Model file for the job. Use its own axes, mm. A direction names the side the tool comes from. Round coordinates to 2 decimals unless told otherwise and drop trailing zeros. Order: outer loops, then holes, each group sorted by start corner. A loop starts at its lowest first (then second) coordinate and runs counter-clockwise, first axis right, second up. Notation, with made-up numbers: M 76.25,30 L 94.25,30 A33 ccw 94.25,69 Z; hole C -32,63 d1. An arc over 180 degrees is marked long. Return JSON: item names as keys, results as strings. Group by question number.
Item 1: Pin check, flat tips, straight feed: pin 1 Ø13 at (x, y) = (18, -36.5) entering from +Z; pin 2 Ø1.5 at (x, z) = (29.5, 12) entering from -Y (3 decimals); pin 3 Ø8 at (x, y) = (10.5, 11) entering from +Z. Stop position of each tip, or through.
Item 2: Slice it at B-B on z = -6. Write the cut outline in (x, y) (3 decimals), then the cut area to 3 significant figures.
Item 3: Pull direction Y, two halves, no side cores. Call faces 4 (the face through (-45.12, -25.07, 6.59)), 5 (the face through (-15, 36.875, -2)), 6 (the face through (-44.425, 8, 9)): pulls with the +Y half, pulls with the -Y half, needs draft (parallel to the pull), parting line crosses it, or undercut.
Item 4: Probe line 1 along X through (y, z) = (34, -4) (3 decimals); line 2 along Z through (x, y) = (-12.5, -16); line 3 along Z through (x, y) = (-10.5, -0.5). List the from-to ranges inside material, lowest first.
Item 5: Slice it at D-D on x = -9. Write the cut outline in (y, z) (3 decimals).
Item 6: Slice it at A-A on y = 7. Write the cut outline in (x, z) (3 decimals), then the cut area to 3 significant figures.
Item 7: Slice it at C-C on x = -31. Write the cut outline in (y, z) (3 decimals).
Item 8: Which spindle directions (+Z, -Z, +X, -X, +Y, -Y) get a long thin tool onto all of the face, cutting with end or side? Do faces 1 (the face through (-42, 29.375, 9)), 2 (the face through (-37, -5.425, -1)), 3 (the face through (21.39, -40.7, 6.28)). Say none if no direction does.
from build123d import *

# Parameters (mm, degrees)
SKETCH1_W                             = 92.75
SKETCH1_H                             = 86.75
SKETCH1_R                             = 1.55
BOSS_EXTRUDE1_FIRST_PCB_DEPTH         = 1.6
SKETCH2_R                             = 6
BOSS_EXTRUDE2_SPEAKER_DEPTH           = 9.5
SKETCH15_R                            = 1.25
CUT_EXTRUDE1_SPEAKER_HOLE_DEPTH       = 5
SKETCH3_W                             = 12
SKETCH3_H                             = 11.65
BOSS_EXTRUDE3_ROTARY_SWITCH_DEPTH     = 4.5
SKETCH4_W                             = 5.83
SKETCH4_H                             = 5.83
BOSS_EXTRUDE4_RESET_SWITCH_DEPTH      = 3.5
SKETCH5_R                             = 1.75
BOSS_EXTRUDE5_RESET_BUTTON_DEPTH      = 0.5
SKETCH16_R                            = 3.415
BOSS_EXTRUDE6_ROTARY_SWITCH_DEPTH     = 7
SKETCH17_R                            = 2.935
BOSS_EXTRUDE7_ROTARY_SWITCH_DEPTH     = 6.4
BOSS_EXTRUDE8_ROTARY_SWITCH_DEPTH     = 6.2
BOSS_EXTRUDE9_SD_CARD_SLOT_DEPTH      = 3
SKETCH19_W                            = 50
SKETCH19_H                            = 2.5
BOSS_EXTRUDE10_CONNECTOR_DEPTH        = 4.2
SKETCH11_W                            = 92.75
SKETCH11_H                            = 70
SKETCH11_R                            = 1.55
BOSS_EXTRUDE11_UPPER_PCB_DEPTH        = 1.6
SKETCH12_W                            = 78.45
SKETCH12_H                            = 51
BOSS_EXTRUDE12_LCD_DEPTH              = 8.3
SKETCH24_W                            = 5.4
SKETCH24_H                            = 43
BOSS_EXTRUDE13_LCD_BUMPOUT_DEPTH      = 3.5
CUT_EXTRUDE2_SCREEN_RECESS_DEPTH      = 1
SKETCH21_W                            = 20.2
SKETCH21_H                            = 8.85
SKETCH21_W_2                          = 18.2
SKETCH21_H_2                          = 6.85
BOSS_EXTRUDE14_CONNECTORS_DEPTH       = 9
SKETCH22_W                            = 18.2
SKETCH22_H                            = 6.85
BOSS_EXTRUDE15_CONNECTOR_RECESS_DEPTH = 2.55
SKETCH23_W                            = 4.4
SKETCH23_H                            = 1
CUT_EXTRUDE3_CONNECTOR_NOTCH_DEPTH    = 6.45
SKETCH20_W                            = 2.153
SKETCH20_H                            = 23.75
BOSS_EXTRUDE16_SD_CARD_DEPTH          = 10.4
FILLET1_SD_CARD_R                     = 1


with BuildPart() as part:
    # Sketch1 → Boss-Extrude1 - First PCB (new body)
    with BuildSketch(Plane.XY):
        Rectangle(SKETCH1_W, SKETCH1_H)
        with Locations((-43.975, 40.975)):
            Circle(SKETCH1_R, mode=Mode.SUBTRACT)
        with Locations((43.975, 40.975)):
            Circle(SKETCH1_R, mode=Mode.SUBTRACT)
        with Locations((43.975, -24.025)):
            Circle(SKETCH1_R, mode=Mode.SUBTRACT)
        with Locations((-43.975, -24.025)):
            Circle(SKETCH1_R, mode=Mode.SUBTRACT)
    extrude(amount=BOSS_EXTRUDE1_FIRST_PCB_DEPTH)

    # Sketch2 → Boss-Extrude2 - Speaker (add)
    with BuildSketch(Plane.XY.offset(1.6)):
        with Locations((18.625, -35.375)):
            Circle(SKETCH2_R)
    extrude(amount=BOSS_EXTRUDE2_SPEAKER_DEPTH)

    # Sketch15 → Cut-Extrude1 - Speaker Hole (cut)
    with BuildSketch(Plane.XY.offset(11.1)):
        with Locations((18.625, -35.375)):
            Circle(SKETCH15_R)
    extrude(amount=-CUT_EXTRUDE1_SPEAKER_HOLE_DEPTH, mode=Mode.SUBTRACT)

    # Sketch3 → Boss-Extrude3 - Rotary Switch (add)
    with BuildSketch(Plane(origin=(0, 0, 1.6), x_dir=(-1, 0, 0), z_dir=(0, 0, 1))):
        with Locations((-36.375, 35.375)):
            Rectangle(SKETCH3_W, SKETCH3_H)
    extrude(amount=BOSS_EXTRUDE3_ROTARY_SWITCH_DEPTH)

    # Sketch4 → Boss-Extrude4 - Reset Switch (add)
    with BuildSketch(Plane(origin=(0, 0, 1.6), x_dir=(-1, 0, 0), z_dir=(0, 0, 1))):
        with Locations((-3.375, 35.375)):
            Rectangle(SKETCH4_W, SKETCH4_H)
    extrude(amount=BOSS_EXTRUDE4_RESET_SWITCH_DEPTH)

    # Sketch5 → Boss-Extrude5 - Reset Button (add)
    with BuildSketch(Plane(origin=(0, 0, 5.1), x_dir=(-1, 0, 0), z_dir=(0, 0, 1))):
        with Locations((-3.375, 35.375)):
            Circle(SKETCH5_R)
    extrude(amount=BOSS_EXTRUDE5_RESET_BUTTON_DEPTH)

    # Sketch16 → Boss-Extrude6 - Rotary Switch (add)
    with BuildSketch(Plane.XY.offset(6.1)):
        with Locations((36.375, -35.375)):
            Circle(SKETCH16_R)
    extrude(amount=BOSS_EXTRUDE6_ROTARY_SWITCH_DEPTH)

    # Sketch17 → Boss-Extrude7 - Rotary Switch (add)
    with BuildSketch(Plane.XY.offset(13.1)):
        with Locations((36.375, -35.375)):
            Circle(SKETCH17_R)
    extrude(amount=BOSS_EXTRUDE7_ROTARY_SWITCH_DEPTH)

    # Sketch18 → Boss-Extrude8 - Rotary Switch (add)
    with BuildSketch(Plane.XY.offset(19.5)):
        with BuildLine():
            Line((33.831773703, -33.91), (38.918226297, -33.91))
            ThreePointArc((38.918226297, -33.91), (36.375, -38.31), (33.831773703, -33.91))
        make_face()
    extrude(amount=BOSS_EXTRUDE8_ROTARY_SWITCH_DEPTH)

    # Sketch9 → Boss-Extrude9 - SD Card Slot (add)
    with BuildSketch(Plane(origin=(0, 0, 0), x_dir=(1, 0, 0), z_dir=(0, 0, -1))):
        Polygon((-46.125, 5.425), (-27.875, 5.425), (-25.875, 3.425), (-20.375, 3.425), (-20.375, -20.975), (-46.125, -20.975), align=None)
    extrude(amount=BOSS_EXTRUDE9_SD_CARD_SLOT_DEPTH)

    # Sketch19 → Boss-Extrude10 - Connector (add)
    with BuildSketch(Plane.XY.offset(1.6)):
        with Locations((-8.375, -24.125)):
            Rectangle(SKETCH19_W, SKETCH19_H)
    extrude(amount=BOSS_EXTRUDE10_CONNECTOR_DEPTH)

    # Sketch11 → Boss-Extrude11 - Upper PCB (add)
    with BuildSketch(Plane(origin=(0, -2, 5.8), x_dir=(1, 0, 0), z_dir=(0, 0, -1))):
        with Locations((0, -10.375)):
            Rectangle(SKETCH11_W, SKETCH11_H)
        with Locations((-43.975, -42.975)):
            Circle(SKETCH11_R, mode=Mode.SUBTRACT)
        with Locations((-43.975, 22.025)):
            Circle(SKETCH11_R, mode=Mode.SUBTRACT)
        with Locations((43.975, -42.975)):
            Circle(SKETCH11_R, mode=Mode.SUBTRACT)
        with Locations((43.975, 22.025)):
            Circle(SKETCH11_R, mode=Mode.SUBTRACT)
    extrude(amount=-BOSS_EXTRUDE11_UPPER_PCB_DEPTH)

    # Sketch12 → Boss-Extrude12 - LCD (add)
    with BuildSketch(Plane(origin=(0, 0, 7.4), x_dir=(-1, 0, 0), z_dir=(0, 0, 1))):
        with Locations((-0.2, -8.475)):
            Rectangle(SKETCH12_W, SKETCH12_H)
    extrude(amount=BOSS_EXTRUDE12_LCD_DEPTH)

    # Sketch24 → Boss-Extrude13 - LCD Bumpout (add)
    with BuildSketch(Plane.XY.offset(7.4)):
        with Locations((-41.725, 7.875)):
            Rectangle(SKETCH24_W, SKETCH24_H)
    extrude(amount=BOSS_EXTRUDE13_LCD_BUMPOUT_DEPTH)

    # Sketch13 → Cut-Extrude2 - Screen Recess (cut)
    with BuildSketch(Plane(origin=(0, 0, 15.7), x_dir=(-1, 0, 0), z_dir=(0, 0, 1))):
        with BuildLine():
            Line((-34.2, 11.525), (33.8, 11.525))
            ThreePointArc((33.8, 11.525), (35.214213562, 10.939213562), (35.8, 9.525))
            Line((35.8, 9.525), (35.8, -26.475))
            ThreePointArc((35.8, -26.475), (35.214213562, -27.889213562), (33.8, -28.475))
            Line((33.8, -28.475), (-34.2, -28.475))
            ThreePointArc((-34.2, -28.475), (-35.614213562, -27.889213562), (-36.2, -26.475))
            Line((-36.2, -26.475), (-36.2, 9.525))
            ThreePointArc((-36.2, 9.525), (-35.614213562, 10.939213562), (-34.2, 11.525))
        make_face()
    extrude(amount=-CUT_EXTRUDE2_SCREEN_RECESS_DEPTH, mode=Mode.SUBTRACT)

    # Sketch21 → Boss-Extrude14 - Connectors (add)
    with BuildSketch(Plane(origin=(0, 0, 0), x_dir=(-1, 0, 0), z_dir=(0, 0, -1))):
        with Locations((-15.525, 32.45)):
            Rectangle(SKETCH21_W, SKETCH21_H)
        with Locations((-15.525, 32.45)):
            Rectangle(SKETCH21_W_2, SKETCH21_H_2, mode=Mode.SUBTRACT)
        with Locations((14.975, 32.45)):
            Rectangle(SKETCH21_W, SKETCH21_H)
        with Locations((14.975, 32.45)):
            Rectangle(SKETCH21_W_2, SKETCH21_H_2, mode=Mode.SUBTRACT)
    extrude(amount=BOSS_EXTRUDE14_CONNECTORS_DEPTH)

    # Sketch22 → Boss-Extrude15 - Connector Recess (add)
    with BuildSketch(Plane(origin=(0, 0, 0), x_dir=(-1, 0, 0), z_dir=(0, 0, -1))):
        with Locations((-15.525, 32.45)):
            Rectangle(SKETCH22_W, SKETCH22_H)
        with Locations((14.975, 32.45)):
            Rectangle(SKETCH22_W, SKETCH22_H)
    extrude(amount=BOSS_EXTRUDE15_CONNECTOR_RECESS_DEPTH)

    # Sketch23 → Cut-Extrude3 - Connector Notch (cut)
    with BuildSketch(Plane(origin=(0, 0, -9), x_dir=(-1, 0, 0), z_dir=(0, 0, -1))):
        with Locations((-15.525, 36.375)):
            Rectangle(SKETCH23_W, SKETCH23_H)
        with Locations((14.975, 36.375)):
            Rectangle(SKETCH23_W, SKETCH23_H)
    extrude(amount=-CUT_EXTRUDE3_CONNECTOR_NOTCH_DEPTH, mode=Mode.SUBTRACT)

    # Sketch20 → Boss-Extrude16 - SD Card (add)
    with BuildSketch(Plane.ZY.offset(46.125)):
        with Locations((-1.3465, 7.775)):
            Rectangle(SKETCH20_W, SKETCH20_H)
    extrude(amount=BOSS_EXTRUDE16_SD_CARD_DEPTH)

    # Fillet1 - SD Card
    fillet1_sd_card_edges = [part.edges().sort_by_distance(p)[0] for p in [
        (-56.525, -4.1, -1.3465),
        (-56.525, 19.65, -1.3465),
    ]]
    fillet(fillet1_sd_card_edges, radius=FILLET1_SD_CARD_R)


solid = part.part
Output values:
{
 "1": {"pin 1": "z = 11.1", "pin 2": "y = -17.025", "pin 3": "z = 14.7"},
 "2": {"outline": "M -25.075,28.025 L -4.875,28.025 L -4.875,36.875 L -12.775,36.875 L -12.775,35.875 L -5.875,35.875 L -5.875,29.025 L -24.075,29.025 L -24.075,35.875 L -17.175,35.875 L -17.175,36.875 L -25.075,36.875 Z; M 5.425,28.025 L 25.625,28.025 L 25.625,36.875 L 17.725,36.875 L 17.725,35.875 L 24.625,35.875 L 24.625,29.025 L 6.425,29.025 L 6.425,35.875 L 13.325,35.875 L 13.325,36.875 L 5.425,36.875 Z", "area": "99.4 mm²"},
 "3": {"face 4": "undercut", "face 5": "pulls with the +Y half", "face 6": "needs draft"},
 "4": {"line 1": "-25.075 to -24.075, -5.875 to -4.875, 5.425 to 6.425, 24.625 to 25.625", "line 2": "0 to 1.6, 5.8 to 15.7", "line 3": "0 to 1.6, 5.8 to 14.7"},
 "5": {"outline": "M -43.375,0 L 28.025,0 L 28.025,-9 L 29.025,-9 L 29.025,-2.55 L 35.875,-2.55 L 35.875,-9 L 36.875,-9 L 36.875,0 L 43.375,0 L 43.375,1.6 L -22.875,1.6 L -22.875,5.8 L 43.375,5.8 L 43.375,7.4 L 33.975,7.4 L 33.975,15.7 L 28.475,15.7 L 28.475,14.7 L -11.525,14.7 L -11.525,15.7 L -17.025,15.7 L -17.025,7.4 L -26.625,7.4 L -26.625,5.8 L -25.375,5.8 L -25.375,1.6 L -43.375,1.6 Z"},
 "6": {"outline": "M -56.525,-2.423 L -46.125,-2.423 L -46.125,-3 L -20.375,-3 L -20.375,0 L 46.375,0 L 46.375,1.6 L -46.375,1.6 L -46.375,0 L -46.125,0 L -46.125,-0.27 L -56.525,-0.27 Z; M -46.375,5.8 L 46.375,5.8 L 46.375,7.4 L 39.425,7.4 L 39.425,15.7 L 36.2,15.7 L 36.2,14.7 L -35.8,14.7 L -35.8,15.7 L -39.025,15.7 L -39.025,10.9 L -44.425,10.9 L -44.425,7.4 L -46.375,7.4 Z", "area": "994 mm²"},
 "7": {"outline": "M -43.375,0 L -5.425,0 L -5.425,-3 L 20.975,-3 L 20.975,0 L 43.375,0 L 43.375,1.6 L -22.875,1.6 L -22.875,5.8 L 43.375,5.8 L 43.375,7.4 L 33.975,7.4 L 33.975,15.7 L 28.475,15.7 L 28.475,14.7 L -11.525,14.7 L -11.525,15.7 L -17.025,15.7 L -17.025,7.4 L -26.625,7.4 L -26.625,5.8 L -25.375,5.8 L -25.375,1.6 L -43.375,1.6 Z"},
 "8": {"face 1": "+Z, -X, +Y", "face 2": "-Z, +X, -X, -Y", "face 3": "+Z"}
}
